```python
from build123d import *

# Parameters (mm, degrees)
CROQUIS2_W              = 136.848636308
CROQUIS2_H              = 84.76602742
SALIENTE_EXTRUIR1_DEPTH = 15
CORTAR_EXTRUIR1_START   = 15
CORTAR_EXTRUIR1_DEPTH   = 27
CROQUIS4_W              = 82.76602742
CROQUIS4_H              = 134.848636308
CORTAR_EXTRUIR2_DEPTH   = 15
CROQUIS6_R              = 1.5
CORTAR_EXTRUIR3_DEPTH   = 10


with BuildPart() as part:
    # Croquis2 → Saliente-Extruir1 (new, symmetric)
    with BuildSketch(Plane(origin=(0, 0, 0), x_dir=(0, 1, 0), z_dir=(0, 0, 1))):
        Rectangle(CROQUIS2_W, CROQUIS2_H)
    extrude(amount=SALIENTE_EXTRUIR1_DEPTH, both=True)

    # Croquis3 → Cortar-Extruir1 (cut)
    with BuildSketch(Plane(origin=(0, 0, 0), x_dir=(0, 1, 0), z_dir=(0, 0, 1)).offset(CORTAR_EXTRUIR1_START)):
        Polygon((-55.424318154, -39.38301371), (-47.845299462, -39.38301371), (-49, -41.38301371), (-41, -41.38301371), (-42.154700538, -39.38301371), (42.154700538, -39.38301371), (41, -41.38301371), (49, -41.38301371), (47.845299462, -39.38301371), (55.424318154, -39.38301371), (65.424318154, -29.38301371), (65.424318154, -17.845299462), (67.424318154, -19), (67.424318154, -11), (65.424318154, -12.154700538), (65.424318154, 12.154700538), (67.424318154, 11), (67.424318154, 19), (65.424318154, 17.845299462), (65.424318154, 29.38301371), (55.424318154, 39.38301371), (47.845299462, 39.38301371), (49, 37.38301371), (41, 37.38301371), (42.154700538, 39.38301371), (-42.154700538, 39.38301371), (-41, 37.38301371), (-49, 37.38301371), (-47.845299462, 39.38301371), (-55.424318154, 39.38301371), (-65.424318154, 29.38301371), (-65.424318154, 17.845299462), (-63.424318154, 19), (-63.424318154, 11), (-65.424318154, 12.154700538), (-65.424318154, -12.154700538), (-63.424318154, -11), (-63.424318154, -19), (-65.424318154, -17.845299462), (-65.424318154, -29.38301371), align=None)
    extrude(amount=-CORTAR_EXTRUIR1_DEPTH, mode=Mode.SUBTRACT)

    # Croquis4 → Cortar-Extruir2 (cut)
    with BuildSketch(Plane.XY.offset(15)):
        Rectangle(CROQUIS4_W, CROQUIS4_H)
    extrude(amount=-CORTAR_EXTRUIR2_DEPTH, mode=Mode.SUBTRACT)

    # Croquis6 → Cortar-Extruir3 (cut)
    with BuildSketch(Plane.XY):
        with Locations(Location((-37, 63, 0), (0, 0, 180))):
            Circle(CROQUIS6_R)
        with Locations(Location((37, 63, 0), (0, 0, 180))):
            Circle(CROQUIS6_R)
        with Locations(Location((37, -63, 0), (0, 0, 180))):
            Circle(CROQUIS6_R)
        with Locations(Location((-37, -63, 0), (0, 0, 180))):
            Circle(CROQUIS6_R)
    extrude(amount=-CORTAR_EXTRUIR3_DEPTH, mode=Mode.SUBTRACT)


solid = part.part
```
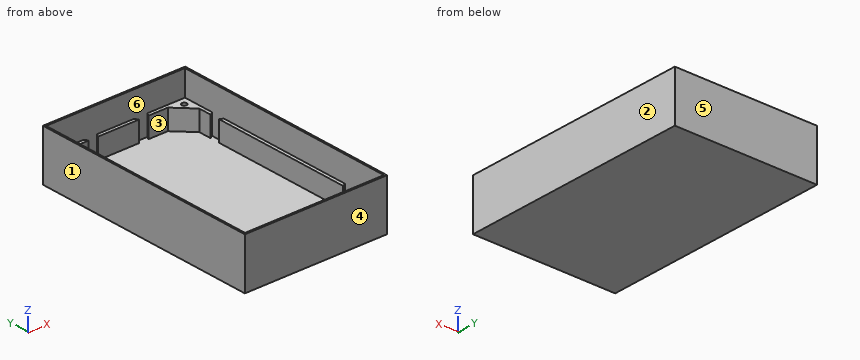
Can you work these out from the model? Positions are in its coordinate system, mm. Face numbers are marked on the shaded views. A direction names the side the tool comes from. Round coordinates to 2 decimals unless told otherwise and drop trailing zeros. Order: outer loops, then holes, each group sorted by start corner. A loop starts at its lowest first (then second) coordinate and runs counter-clockwise, first axis right, second up. Notation, with made-up numbers: (12.5, 60) -> (36.5, 60) arc R16 cw to (36.5, 77) -> close; hole circle Ø5 at (65, 70). An arc over 180 degrees is marked (long way). Return JSON: item names as keys, results as strings. Group by question number.
1. If we section it at A-A, the plane y = 9.5: Write out the boundary of the cut face in (x, z).
2. Will these pins go through, and if not, where does the flat tip stop? pin 1 (8 mm diameter, centred on x = -3, y = -14.5, fed in from +Z); pin 2 (2.5 mm diameter, centred on x = -37, y = 62.5, fed in from +Z); pin 3 (0.9 mm diameter, centred on x = -36.5, y = -63, fed in from +Z).
3. Which directions (+Z, -Z, +X, -X, +Y, -Y) give clear straight access to the entire face, cutting with the end or side of a thin tool? Please do the marked faces 5 and 6.
4. If we section it at C-C, the plane y = 63: Write out the boundary of the cut face in (x, z), then the cut area to 3 significant figures.
5. If we section it at B-B, the plane x = -27: Write out the boundary of the cut face in (y, z), then the cut area to 3 significant figures.
6. I need wall thicknesses on line 1 (X direction, y = -6, z = -4.75); line 2 (X direction, y = 44, z = 0.5); line 3 (Y direction, x = -19, z = 4.25). Which ranges of each line are inside material? Lowest first, please. Write a range as [from, to].
7. We'd pull the mould along X, two halves only. Please class the marked faces 1, 2, 3 and 4: released by +X, released by -X, zero draft, split by the parting line, or undercut.
8. If we section it at D-D, the plane x = 37: Write out the boundary of the cut face in (y, z), then the cut area to 3 significant figures.
Output values:
{
 "1": {"outline": "(-42.38, -15) -> (42.38, -15) -> (42.38, 15) -> (41.38, 15) -> (41.38, 0) -> (39.38, 0) -> (39.38, -12) -> (-39.38, -12) -> (-39.38, 0) -> (-41.38, 0) -> (-41.38, 15) -> (-42.38, 15) -> close"},
 "2": {"pin 1": "z = -12", "pin 2": "z = 0", "pin 3": "z = -10"},
 "3": {"face 5": "+Z, -Z, +X, -X, +Y", "face 6": "+Z"},
 "4": {"outline": "(-42.38, -15) -> (42.38, -15) -> (42.38, 15) -> (41.38, 15) -> (41.38, 0) -> (38.5, 0) -> (38.5, -10) -> (35.5, -10) -> (35.5, 0) -> (31.81, 0) -> (31.81, -12) -> (-31.81, -12) -> (-31.81, 0) -> (-35.5, 0) -> (-35.5, -10) -> (-38.5, -10) -> (-38.5, 0) -> (-41.38, 0) -> (-41.38, 15) -> (-42.38, 15) -> close", "area": "478 mm²"},
 "5": {"outline": "(-68.42, -15) -> (68.42, -15) -> (68.42, 15) -> (67.42, 15) -> (67.42, 0) -> (65.42, 0) -> (65.42, -12) -> (-65.42, -12) -> (-65.42, 0) -> (-67.42, 0) -> (-67.42, 15) -> (-68.42, 15) -> close", "area": "513 mm²"},
 "6": {"line 1": "[-42.38, -39.38], [39.38, 42.38]", "line 2": "[-42.38, -41.38], [41.38, 42.38]", "line 3": "[-68.42, -67.42], [67.42, 68.42]"},
 "7": {"face 1": "released by -X", "face 2": "released by +X", "face 3": "undercut", "face 4": "zero draft"},
 "8": {"outline": "(-68.42, -15) -> (68.42, -15) -> (68.42, 15) -> (67.42, 15) -> (67.42, 0) -> (64.5, 0) -> (64.5, -10) -> (61.5, -10) -> (61.5, 0) -> (57.81, 0) -> (57.81, -12) -> (-57.81, -12) -> (-57.81, 0) -> (-61.5, 0) -> (-61.5, -10) -> (-64.5, -10) -> (-64.5, 0) -> (-67.42, 0) -> (-67.42, 15) -> (-68.42, 15) -> close", "area": "635 mm²"}
}
